Read the model definition and answer for the solid it produces. Units are mm, in the model's axes. Face numbers are marked on the shaded views. A direction names the side the tool comes from. Coordinates: 2 decimals unless noted, no trailing zeros. Loops run counter-clockwise (first coordinate to the right, second up) from the corner with the lowest first, then second, coordinate; pieces in that order, holes last. Notation, with made-up numbers: (-19.5, 42) - (27.5, 42) arc R31 cw to (27.5, 77) - close; hole circle Ø4 at (2, 18). An arc over 180 degrees is marked (long way). Use one line per item in the form item = value. Start each with the question number.
1) The mould has two halves that part along X. Classify the marked faces 5, 6 and 7: released by +X, released by -X, zero draft, split by the parting line, or undercut.
2) A cutting plane is placed at A-A (y = 0). Give the vertices of the cut face in (x, z).
3) A cutting plane is placed at B-B (x = 0). Give the vertices of the cut face in (y, z), and give its area (3 significant figures).
4) A cutting plane is placed at C-C (z = 4.5). Give the vertices of the cut face in (x, y).
5) Which of the six approach directions +Z, -Z, +X, -X, +Y, -Y give full straight-line access (tool end or side, diameter ignored) to the marked faces 1, 2, 3 and 4?
6) Consider line 1 (Z direction, x = 0.5, y = 0.5); line 2 (X direction, y = -14, z = 27.5); line 3 (Y direction, x = 14, z = 6). Determine where each line is inside the solid, lowest interval first.
7) A cutting plane is placed at D-D (z = 22). Give the vertices of the cut face in (x, y) (3 decimals).
8) Each of these flat-tipped pins is pushed along its axis until it touches: P1, Ø9, axis at y = 1.5, z = 19, coming from the +X side; P2, Ø4, axis at x = 27, z = 5, coming from the -Y side; P3, Ø1.5, axis at y = 2, z = 19, coming from the -X side. Where does it stop, or does it pass through?
Autodesk Inventor part; units mm, degrees
ref_plane "YZ Plane" through (0, 0, 0) normal (1, 0, 0) x (0, 1, 0)
ref_plane "XZ Plane" through (0, 0, 0) normal (0, 1, 0) x (-1, 0, 0)
ref_plane "XY Plane" through (0, 0, 0) normal (0, 0, 1) x (1, 0, 0)
sketch "草图1" plane through (0, 0, 0) normal (0, 0, 1) x (1, 0, 0)
  line L0 (-30, 15) -> (30, 15)
  line L1 (30, -15) -> (-30, -15)
  line L2 (-30, 15) -> (30, -15) construction
  line L3 (30, 15) -> (-30, -15) construction
  arc A0 (-22, -5) -> (-22, 5) centre (-22, 0) ccw
  line L4 (-22, 5) -> (-30, 5)
  line L5 (-22, -5) -> (-30, -5)
  line L6 (-30, -15) -> (-30, -5)
  line L7 (-30, 5) -> (-30, 15)
  arc A1 (22, 5) -> (22, -5) centre (22, 0) ccw
  line L8 (22, 5) -> (30, 5)
  line L9 (22, -5) -> (30, -5)
  line L10 (30, 15) -> (30, 5)
  line L11 (30, -5) -> (30, -15)
  point P0 (0, 0)
  dimension "d0" = 60
  dimension "d1" = 30
  dimension "d3" = 10
  dimension "d5" = 10
extrude "拉伸1" add sketch "草图1" along normal blind 9
sketch "草图2" plane through (-30, -15, 0) normal (0, -1, 0) x (1, 0, 0)
  line L0 (30, 0) -> (30, 27)
  circle A0 centre (30, 27) radius 8
  circle A1 centre (30, 27) radius 14
  line L1 (60, 9) -> (0, 9)
  line L2 (44, 27) -> (44, 9)
  line L3 (16, 27) -> (16, 9)
  dimension "d8" = 27
  dimension "d9" = 16
  dimension "d10" = 28
extrude "拉伸2" add sketch "草图2" against normal blind 30
sketch "草图3" plane through (-30, -15, 0) normal (0, -1, 0) x (1, 0, 0)
  line L0 (30, 0) -> (30, 27)
  circle A0 centre (30, 27) radius 14
  circle A1 centre (30, 27) radius 8
  dimension "d13" = 27
  dimension "d14" = 28
  dimension "d15" = 16
extrude "拉伸3" add sketch "草图3" along normal blind 5
properties part number "2-5"
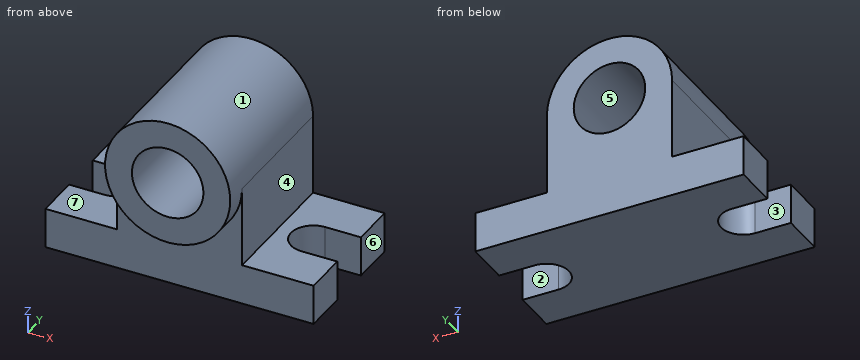
Found:
q1.face_5 = undercut
q1.face_6 = released by +X
q1.face_7 = zero draft
q2.outline = (-17, 0) - (17, 0) - (17, 9) - (14, 9) - (14, 27) arc R14 ccw to (-14, 27) - (-14, 9) - (-17, 9) - close; hole circle Ø16 at (0, 27)
q3.outline = (-20, 13) - (-15, 13) - (-15, 0) - (15, 0) - (15, 19) - (-20, 19) - close; (-20, 35) - (15, 35) - (15, 41) - (-20, 41) - close
q3.area = 810 mm^2
q4.outline = (-30, -15) - (30, -15) - (30, -5) - (22, -5) arc R5 cw to (22, 5) - (30, 5) - (30, 15) - (-30, 15) - (-30, 5) - (-22, 5) arc R5 cw to (-22, -5) - (-30, -5) - close
q5.face_1 = -Y
q5.face_2 = +Z, -Z, +X
q5.face_3 = +Z, -Z, -X
q5.face_4 = +Z, +X, +Y, -Y
q6.line_1 = 0 to 19.02, 34.98 to 40.99
q6.line_2 = -13.99 to -7.98, 7.98 to 13.99
q6.line_3 = -15 to 15
q7.outline = (-14, -15) - (-13.077, -15) - (-13.077, -20) - (-6.245, -20) - (-6.245, 15) - (-14, 15) - close; (6.245, -20) - (13.077, -20) - (13.077, -15) - (14, -15) - (14, 15) - (6.245, 15) - close
q8.P1 = 14
q8.P2 = -15
q8.P3 = -14
